```python
from build123d import *

# Parameters (mm, degrees)
BOSS_EXTRUDE1_DEPTH                          = 10
FILLET1_R                                    = 10
SKETCH2_R                                    = 1.75
CUT_EXTRUDE1_DEPTH                           = 10
CBORE_FOR_M4_HEX_SOCKET_HEAD_CAP_SCR_2_COUNT = 2
CBORE_FOR_M4_HEX_SOCKET_HEAD_CAP_SCR_2_PITCH = 10
CBORE_FOR_M4_HEX_SOCKET_HEAD_CAP_SCR_3_COUNT = 2
CBORE_FOR_M4_HEX_SOCKET_HEAD_CAP_SCR_3_PITCH = 60
CBORE_FOR_M4_HEX_SOCKET_HEAD_CAP_SCR_4_COUNT = 2
CBORE_FOR_M4_HEX_SOCKET_HEAD_CAP_SCR_4_PITCH = 152.099474029
CBORE_FOR_M4_HEX_SOCKET_HEAD_CAP_SCR_5_COUNT = 2
CBORE_FOR_M4_HEX_SOCKET_HEAD_CAP_SCR_5_PITCH = 161.939031737
CBORE_FOR_M4_HEX_SOCKET_HEAD_CAP_SCR_6_COUNT = 2
CBORE_FOR_M4_HEX_SOCKET_HEAD_CAP_SCR_6_PITCH = 162.67836365
CBORE_FOR_M4_HEX_SOCKET_HEAD_CAP_SCR_7_COUNT = 2
CBORE_FOR_M4_HEX_SOCKET_HEAD_CAP_SCR_7_PITCH = 152.886395732
CBORE_FOR_M4_HEX_SOCKET_HEAD_CAP_SCR_8_COUNT = 2
CBORE_FOR_M4_HEX_SOCKET_HEAD_CAP_SCR_8_PITCH = 60.827625303
FILLET2_R                                    = 2.5
FILLET3_R                                    = 2.5
SKETCH5_W                                    = 43
SKETCH5_H                                    = 121
BOSS_EXTRUDE2_DEPTH                          = 20
CHAMFER1_SIZE                                = 20
SKETCH6_R                                    = 3.462541839
CUT_EXTRUDE2_DEPTH                           = 20
SKETCH7_R                                    = 2.25
CUT_EXTRUDE3_DEPTH                           = 20
FILLET4_R                                    = 5


# Some blends are built 0.0001 mm under size
with BuildPart() as part:
    # Sketch1 → Boss-Extrude1 (new body)
    with BuildSketch(Plane(origin=(0, 0, 0), x_dir=(1, 0, 0), z_dir=(0, 1, 0))):
        Polygon((-21.5, -89), (21.5, -89), (21.5, 70.5), (53.5, 70.5), (53.5, 89), (-21.5, 89), (-21.5, -70.5), (-53.5, -70.5), (-53.5, -89), align=None)
    extrude(amount=BOSS_EXTRUDE1_DEPTH)

    # Fillet1
    fillet1_edges = [part.edges().sort_by_distance(p)[0] for p in [
        (-21.5, 5, 70.5),
        (-21.5, 5, -89),
        (21.5, 5, -70.5),
        (21.5, 5, 89),
    ]]
    fillet(fillet1_edges, radius=FILLET1_R)

    # Sketch2 → Cut-Extrude1 (cut)
    with BuildSketch(Plane(origin=(0, 10, 0), x_dir=(1, 0, 0), z_dir=(0, 1, 0))):
        with Locations(Location((-14, 74.75, 0), (0, 0, 270))):
            Circle(SKETCH2_R)
        with Locations(Location((-14, 84.75, 0), (0, 0, 270))):
            Circle(SKETCH2_R)
        with Locations(Location((46, 74.75, 0), (0, 0, 270))):
            Circle(SKETCH2_R)
        with Locations(Location((46, 84.75, 0), (0, 0, 270))):
            Circle(SKETCH2_R)
        with Locations(Location((-46, -74.75, 0), (0, 0, 270))):
            Circle(SKETCH2_R)
        with Locations(Location((-46, -84.75, 0), (0, 0, 270))):
            Circle(SKETCH2_R)
        with Locations(Location((14, -74.75, 0), (0, 0, 270))):
            Circle(SKETCH2_R)
        with Locations(Location((14, -84.75, 0), (0, 0, 270))):
            Circle(SKETCH2_R)
    extrude(amount=-CUT_EXTRUDE1_DEPTH, mode=Mode.SUBTRACT)

    # Sketch4 → CBORE for M4 Hex Socket Head Cap Screw1 (revolve, cut)
    with BuildSketch(Plane(origin=(-14, 10, -74.75), x_dir=(0, 0, 1), z_dir=(1, 0, 0))):
        Polygon((0, 0), (0, 11.351936393), (2.25, 10), (2.25, 4.4), (4, 4.4), (4, 0.025), (4.025, 0), align=None)
    cbore_for_m4_hex_socket_head_cap_screw1 = revolve(axis=Axis((-14, 16.35, -74.75), (0, -1, 0)), mode=Mode.SUBTRACT)

    # CBORE for M4 Hex Socket Head Cap Scr 2: CBORE for M4 Hex Socket Head Cap Screw1 ×2
    with Locations(*[(0, 0, -i * CBORE_FOR_M4_HEX_SOCKET_HEAD_CAP_SCR_2_PITCH) for i in range(1, CBORE_FOR_M4_HEX_SOCKET_HEAD_CAP_SCR_2_COUNT)]):
        add(cbore_for_m4_hex_socket_head_cap_screw1, mode=Mode.SUBTRACT)

    # CBORE for M4 Hex Socket Head Cap Scr 3: CBORE for M4 Hex Socket Head Cap Screw1 ×2
    with Locations(*[(i * CBORE_FOR_M4_HEX_SOCKET_HEAD_CAP_SCR_3_PITCH, 0, 0) for i in range(1, CBORE_FOR_M4_HEX_SOCKET_HEAD_CAP_SCR_3_COUNT)]):
        add(cbore_for_m4_hex_socket_head_cap_screw1, mode=Mode.SUBTRACT)

    # CBORE for M4 Hex Socket Head Cap Scr 4: CBORE for M4 Hex Socket Head Cap Screw1 ×2
    with Locations(*[Vector(0.1840900514527529, 0, 0.9829093818639248) * (i * CBORE_FOR_M4_HEX_SOCKET_HEAD_CAP_SCR_4_PITCH) for i in range(1, CBORE_FOR_M4_HEX_SOCKET_HEAD_CAP_SCR_4_COUNT)]):
        add(cbore_for_m4_hex_socket_head_cap_screw1, mode=Mode.SUBTRACT)

    # CBORE for M4 Hex Socket Head Cap Scr 5: CBORE for M4 Hex Socket Head Cap Screw1 ×2
    with Locations(*[Vector(0.1729045783441913, 0, 0.9849385802107751) * (i * CBORE_FOR_M4_HEX_SOCKET_HEAD_CAP_SCR_5_PITCH) for i in range(1, CBORE_FOR_M4_HEX_SOCKET_HEAD_CAP_SCR_5_COUNT)]):
        add(cbore_for_m4_hex_socket_head_cap_screw1, mode=Mode.SUBTRACT)

    # CBORE for M4 Hex Socket Head Cap Scr 6: CBORE for M4 Hex Socket Head Cap Screw1 ×2
    with Locations(*[Vector(-0.19670716671795496, 0, 0.9804622841097942) * (i * CBORE_FOR_M4_HEX_SOCKET_HEAD_CAP_SCR_6_PITCH) for i in range(1, CBORE_FOR_M4_HEX_SOCKET_HEAD_CAP_SCR_6_COUNT)]):
        add(cbore_for_m4_hex_socket_head_cap_screw1, mode=Mode.SUBTRACT)

    # CBORE for M4 Hex Socket Head Cap Scr 7: CBORE for M4 Hex Socket Head Cap Screw1 ×2
    with Locations(*[Vector(-0.20930573872668637, 0, 0.9778502481137263) * (i * CBORE_FOR_M4_HEX_SOCKET_HEAD_CAP_SCR_7_PITCH) for i in range(1, CBORE_FOR_M4_HEX_SOCKET_HEAD_CAP_SCR_7_COUNT)]):
        add(cbore_for_m4_hex_socket_head_cap_screw1, mode=Mode.SUBTRACT)

    # CBORE for M4 Hex Socket Head Cap Scr 8: CBORE for M4 Hex Socket Head Cap Screw1 ×2
    with Locations(*[Vector(0.9863939238321426, 0, -0.1643989873053641) * (i * CBORE_FOR_M4_HEX_SOCKET_HEAD_CAP_SCR_8_PITCH) for i in range(1, CBORE_FOR_M4_HEX_SOCKET_HEAD_CAP_SCR_8_COUNT)]):
        add(cbore_for_m4_hex_socket_head_cap_screw1, mode=Mode.SUBTRACT)

    # Fillet2
    # the kernel refuses this fillet: 2.5 mm, written as the material it takes off along each edge
    with BuildSketch(Plane(origin=(-13.754801439, 5.6, -88.742477635), x_dir=(0.9990847033117879, 0, -0.042775642699985884), z_dir=(0, 1, 0))) as fillet2_piece_1:
        with BuildLine():
            CenterArc((5.91336471, -2.497711758), FILLET2_R, 87.548388178, 105.618498276)
            Line((3.479087926, -3.067182162), (3.235660248, -3.124129202))
            ThreePointArc((3.235660248, -3.124129202), (2.064143441, -1.165399671), (-0.025984683, -0.248645925))
            Line((-0.025984683, -0.248645925), (-0.045899922, 0.245750274))
            ThreePointArc((-0.045899922, 0.245750274), (2.274447223, 0.410607251), (6.030997727, 0.249771176))
            Line((6.030997727, 0.249771176), (6.020303816, 0))
        make_face()
    extrude(amount=19.425759541, mode=Mode.SUBTRACT)
    with BuildSketch(Plane(origin=(-17.087010961, 5.6, -87.293690886), x_dir=(-0.5524220177087732, 0, 0.8335645831911094), z_dir=(0, 1, 0))) as fillet2_piece_2:
        with BuildLine():
            CenterArc((6.697143458, 2.309687979), FILLET2_R, 165.124054411, 127.376595494)
            ThreePointArc((4.280933593, 2.951505625), (2.685480046, 0.685252699), (0, 0))
            ThreePointArc((0, 0), (3.826939119, -0.761248083), (7.653878238, 0))
        make_face()
    extrude(amount=23.509695594, mode=Mode.SUBTRACT)

    # Fillet3
    # the kernel refuses this fillet: 2.5 mm, written as the material it takes off along each edge
    with BuildSketch(Plane(origin=(13.75480144, 5.6, 88.742477635), x_dir=(-0.7777172566996915, 0, -0.6286142446934416), z_dir=(0, 1, 0))) as fillet3_piece_1:
        with BuildLine():
            CenterArc((6.087462048, 2.036971289), FILLET3_R, 128.947957862, 105.618498276)
            Line((4.515926436, 3.98126443), (4.358772875, 4.175693744))
            ThreePointArc((4.358772875, 4.175693744), (1.434562202, 1.812109205), (-0.196946455, 0.153987317))
            Line((-0.196946455, 0.153987317), (0.144939573, -0.203697129))
            ThreePointArc((0.144939573, -0.203697129), (2.319033161, 0.490845938), (4.49312675, -0.203697129))
            Line((4.49312675, -0.203697129), (4.638066322, 0))
        make_face()
    extrude(amount=19.425759541, mode=Mode.SUBTRACT)
    with BuildSketch(Plane(origin=(17.087010961, 5.6, 87.293690886), x_dir=(-0.018344711955799436, 0, -0.9998317216128216), z_dir=(0, 1, 0))) as fillet3_piece_2:
        with BuildLine():
            CenterArc((6.824719559, -1.89989263), FILLET3_R, 130.539588182, 127.376595494)
            ThreePointArc((6.30136363, -4.344498645), (2.718581752, -2.798977477), (0, 0))
            ThreePointArc((0, 0), (2.599893165, -0.960171793), (5.19978633, 0))
        make_face()
    extrude(amount=23.509695594, mode=Mode.SUBTRACT)

    # Sketch5 → Boss-Extrude2 (add)
    with BuildSketch(Plane(origin=(0, 10, 0), x_dir=(1, 0, 0), z_dir=(0, 1, 0))):
        Rectangle(SKETCH5_W, SKETCH5_H)
    extrude(amount=BOSS_EXTRUDE2_DEPTH)

    # Chamfer1
    chamfer1_edges = [part.edges().sort_by_distance(p)[0] for p in [
        (0, 30, -60.5),
        (0, 30, 60.5),
    ]]
    chamfer(chamfer1_edges, length=CHAMFER1_SIZE - 0.0001)  # a hair under: the kernel refuses the full size

    # Sketch6 → Cut-Extrude2 (cut)
    with BuildSketch(Plane(origin=(0, 30, 0), x_dir=(1, 0, 0), z_dir=(0, 1, 0))):
        with Locations(Location((0, 0, 0), (0, 0, 270))):
            Circle(SKETCH6_R)
    extrude(amount=-CUT_EXTRUDE2_DEPTH, mode=Mode.SUBTRACT)

    # Sketch7 → Cut-Extrude3 (cut)
    with BuildSketch(Plane(origin=(0, 30, 0), x_dir=(1, 0, 0), z_dir=(0, 1, 0))):
        with Locations(Location((-12.5, 30, 0), (0, 0, 270))):
            Circle(SKETCH7_R)
        with Locations(Location((12.5, 30, 0), (0, 0, 270))):
            Circle(SKETCH7_R)
        with Locations(Location((12.5, -30, 0), (0, 0, 270))):
            Circle(SKETCH7_R)
        with Locations(Location((-12.5, -30, 0), (0, 0, 270))):
            Circle(SKETCH7_R)
    extrude(amount=-CUT_EXTRUDE3_DEPTH, mode=Mode.SUBTRACT)

    # Fillet4
    fillet4_edges = [part.edges().sort_by_distance(p)[0] for p in [
        (0, 30, 40.5001),
        (0, 30, -40.5001),
    ]]
    fillet(fillet4_edges, radius=FILLET4_R)


solid = part.part
```
Read the model definition and answer for the solid it produces. Units are mm, in the model's axes. A direction names the side the tool comes from. Give positions to 0.01 mm unless a question says otherwise; leave off trailing zeros. Order: outer loops, then holes, each group sorted by start corner. A loop starts at its lowest first (then second) coordinate and runs counter-clockwise, first axis right, second up.
(1) For faces 1 (the cylindrical face through (-13.14, 2.84, -72.67)), 2 (the flat face through (-0.3, 19.4, 51.1)), 3 (the flat face through (-21.5, 15, -8)), 4 (the flat face through (-44, 5.6, 73)), 5 (the flat face through (42, 5, -70.5)), determine the directions among +Z, -Z, +X, -X, +Y, -Y from which every point of the face is accessible in a straight line to the end or side of a thin tool.
(2) Straight lines are drawn through the part: L1, parallel to Z at x = -45, y = 4.5; L2, parallel to X at y = 4.45, z = 84.75; L3, parallel to X at y = 9, z = 8.5. For each, find the intervals that lie inside material, in ascending order.
(3) Find section A-A (x = 46). Give the vertices of the cut face in (y, z) (3 decimals), plus the area to 3 significant figures.
(4) Find section C-C (z = 0). Give the vertices of the cut face in (x, y), plus the area to 3 significant figures.
(5) Given pin 1 (6.5 mm diameter, centred on x = 46, z = -74.75, fed in from -Y); pin 2 (3.5 mm diameter, centred on x = -46, z = 74.75, fed in from -Y); pin 3 (23 mm diameter, centred on x = -1, z = 76.5, fed in from +Y); pin 4 (2.5 mm diameter, centred on x = 47.5, z = -74, fed in from +Y), each flat-ended and moving along its own axis, determine where each tip first touches the part or whether it passes through.
(6) For a pull along X with two mould halves and no side action, classify faces 6 (the flat face through (53.5, 5, -80)), 7 (the flat face through (21, 5, -89)), 8 (the cylindrical face through (19.483, 7.769, 82.857)), 9 (the flat face through (0, 10, 0)) as released by +X, released by -X, zero draft, split by the parting line, or undercut.
(7) Find section D-D (y = 26.5). Give the vertices of the cut face in (x, z).
(8) Find section B-B (y = 3.5). Give the number of separate pieces and of enclosed holes in the cut face, plus the area to 3 significant figures.
Result sheet:
1. face 1: +Y, -Y
1. face 2: +Z, +X, -X, +Y
1. face 3: -Z, -X, +Y, -Y
1. face 4: +Y
1. face 5: +Z, +X, +Y, -Y
2. L1: z = 70.5 to 72.73, 76.77 to 82.73, 86.77 to 89
2. L2: x = -53.5 to -48.25, -43.75 to 11.75, 16.25 to 19.68
2. L3: x = -21.5 to 21.5
3. outline: (0, -89) - (10, -89) - (10, -88.775) - (9.975, -88.75) - (5.6, -88.75) - (5.6, -87) - (0, -87) - close; (0, -82.5) - (5.6, -82.5) - (5.6, -80.75) - (9.975, -80.75) - (10, -80.725) - (10, -78.775) - (9.975, -78.75) - (5.6, -78.75) - (5.6, -77) - (0, -77) - close; (0, -72.5) - (5.6, -72.5) - (5.6, -70.75) - (9.975, -70.75) - (10, -70.725) - (10, -70.5) - (0, -70.5) - close
3. area: 64.2 mm2
4. outline: (-21.5, 0) - (21.5, 0) - (21.5, 30) - (3.46, 30) - (3.46, 10) - (-3.46, 10) - (-3.46, 30) - (-21.5, 30) - close
4. area: 1,150 mm2
5. pin 1: stops at y = 0
5. pin 2: passes through
5. pin 3: stops at y = 10
5. pin 4: stops at y = 5.6
6. face 6: released by +X
6. face 7: zero draft
6. face 8: undercut
6. face 9: undercut
7. outline: (-21.5, -44) - (21.5, -44) - (21.5, 44) - (-21.5, 44) - close; hole circle Ø4.5 at (-12.5, -30); hole circle Ø4.5 at (-12.5, 30); hole circle Ø6.93 at (0, 0); hole circle Ø4.5 at (12.5, -30); hole circle Ø4.5 at (12.5, 30)
8. separate pieces: 1
8. enclosed holes: 8
8. area: 8,710 mm2
